```python
from build123d import *

# Parameters (mm, degrees)
SKETCH1_R           = 4.9
BOSS_EXTRUDE1_DEPTH = 4
SKETCH2_R           = 2
CUT_EXTRUDE1_DEPTH  = 4.8
SKETCH3_OUTSIDE_W   = 14.684
SKETCH3_OUTSIDE_H   = 14.684
CUT_EXTRUDE2_DEPTH  = 2.6
FILLET1_R           = 0.3


with BuildPart() as part:
    # Sketch1 → Boss-Extrude1 (new body)
    with BuildSketch(Plane(origin=(0, 0, 0), x_dir=(1, 0, 0), z_dir=(0, 1, 0))):
        Circle(SKETCH1_R)
    extrude(amount=BOSS_EXTRUDE1_DEPTH)

    # Sketch2 → Cut-Extrude1 (cut)
    with BuildSketch(Plane(origin=(0, 4, 0), x_dir=(1, 0, 0), z_dir=(0, 1, 0))):
        Circle(SKETCH2_R)
    extrude(amount=-CUT_EXTRUDE1_DEPTH, mode=Mode.SUBTRACT)

    # Sketch3 outside → Cut-Extrude2 (cut)
    with BuildSketch(Plane(origin=(0, 4, 0), x_dir=(1, 0, 0), z_dir=(0, 1, 0))):
        Rectangle(SKETCH3_OUTSIDE_W, SKETCH3_OUTSIDE_H)
        Polygon((4.041451884, 0), (2.020725942, 3.5), (-2.020725942, 3.5), (-4.041451884, 0), (-2.020725942, -3.5), (2.020725942, -3.5), align=None, mode=Mode.SUBTRACT)
    extrude(amount=-CUT_EXTRUDE2_DEPTH, mode=Mode.SUBTRACT)

    # Fillet1
    fillet1_edges = [part.edges().sort_by_distance(p)[0] for p in [
        (0, 1.4, 3.5),
        (3.031088913, 1.4, 1.75),
        (3.031088913, 1.4, -1.75),
        (0, 1.4, -3.5),
        (-3.031088913, 1.4, -1.75),
        (-3.031088913, 1.4, 1.75),
        (-4.9, 1.4, 0),
        (-4.9, 0, 0),
        (3.031088913, 4, 1.75),
        (0, 4, 3.5),
        (-3.031088913, 4, 1.75),
        (-3.031088913, 4, -1.75),
        (0, 4, -3.5),
        (3.031088913, 4, -1.75),
        (-2, 0, 0),
        (-2, 4, 0),
    ]]
    fillet(fillet1_edges, radius=FILLET1_R)


solid = part.part
```
CAD build for the part. Positions are in the model's coordinates, mm. A direction names the side the tool comes from. Give positions to 0.01 mm unless a question says otherwise; leave off trailing zeros. Order: outer loops, then holes, each group sorted by start corner. A loop starts at its lowest first (then second) coordinate and runs counter-clockwise, first axis right, second up.
(1) Drill centre lines: L1, parallel to X at y = 1.05, z = 0; L2, parallel to Y at x = 2.5, z = -3.25. Where is each one in solid material? Low to high.
(2) Mould opens along Z. For faces 5 (the cylindrical face through (0, 2, 2)), 6 (the flat face through (-3.43, 1.4, 2.02)), 7 (the cylindrical face through (-1.062, 0.694, 4.783)) say: released by +Z, released by -Z, zero draft, split by the parting line, or undercut.
(3) Flat gauge pins, fed straight in: pin 1 (1.6 mm diameter, centred on x = 0, y = 2.5, fed in from -Z); pin 2 (2 mm diameter, centred on x = -3.5, y = 2.5, fed in from +Z); pin 3 (2 mm diameter, centred on x = -3.5, y = 2.5, fed in from -Z). Where does each tip first touch, or does it go through?
(4) Tool access for faces 1 (the flat face through (-3, 2.7, -1.8)), 2 (the flat face through (3.045, 2.714, -1.726)), 3 (the flat face through (0, 3, -3.5)), 4 (the flat face through (3, 2.7, 1.8)): list every direction of +Z, -Z, +X, -X, +Y, -Y with a clear straight run to the whole face (end or side of a thin tool).
(5) Saw through at A-A, the plane x = 0. Give the cut face in (y, z).
(6) Saw through at B-B, the plane y = 2.3. Give the cut face in (x, z).
Results found:
1. L1: x = -4.9 to -2, 2 to 4.9
1. L2: y = 0 to 1.4
2. face 5: undercut
2. face 6: zero draft
2. face 7: split by the parting line
3. pin 1: stops at z = -3.5
3. pin 2: stops at z = 2.67
3. pin 3: stops at z = -2.67
4. face 1: -Z, -X, +Y
4. face 2: -Z, +X, +Y
4. face 3: -Z, +X, -X, +Y
4. face 4: +Z, +X, +Y
5. outline: (0, -4.6) arc R0.3 ccw to (0.3, -4.9) - (1.1, -4.9) arc R0.3 ccw to (1.4, -4.6) - (1.4, -3.8) arc R0.3 cw to (1.7, -3.5) - (3.7, -3.5) arc R0.3 ccw to (4, -3.2) - (4, -2.3) arc R0.3 ccw to (3.7, -2) - (0.3, -2) arc R0.3 ccw to (0, -2.3) - close; (0, 2.3) arc R0.3 ccw to (0.3, 2) - (3.7, 2) arc R0.3 ccw to (4, 2.3) - (4, 3.2) arc R0.3 ccw to (3.7, 3.5) - (1.7, 3.5) arc R0.3 cw to (1.4, 3.8) - (1.4, 4.6) arc R0.3 ccw to (1.1, 4.9) - (0.3, 4.9) arc R0.3 ccw to (0, 4.6) - close
6. outline: (-4.04, 0) - (-2.02, -3.5) - (2.02, -3.5) - (4.04, 0) - (2.02, 3.5) - (-2.02, 3.5) - close; hole circle Ø4 at (0, 0)
